```python
from build123d import *

# Parameters (mm, degrees)
F0_R     = 2.5
F0_R_2   = 8
F0_W     = 5
F0_H     = 9.9
F1_DEPTH = 3.5


with BuildPart() as f1:
    # F0 (on Top) → F1 (new body)
    with BuildSketch(Plane.XY):
        with BuildLine():
            ThreePointArc((0, -5), (-1.464466, -1.464466), (-5, 0))
            Line((-5, 0), (-125.9, 0))
            ThreePointArc((-125.9, 0), (-129.435534, -1.464466), (-130.9, -5))
            Line((-130.9, -5), (-130.9, -25))
            ThreePointArc((-130.9, -25), (-129.435534, -28.535534), (-125.9, -30))
            Line((-125.9, -30), (-5, -30))
            ThreePointArc((-5, -30), (-1.464466, -28.535534), (0, -25))
            Line((0, -25), (0, -5))
        make_face()
        with Locations((-96.3, -25.5)):
            Circle(F0_R, mode=Mode.SUBTRACT)
        with Locations((-76.3, -25.5)):
            Circle(F0_R, mode=Mode.SUBTRACT)
        with Locations((-56.3, -25.5)):
            Circle(F0_R, mode=Mode.SUBTRACT)
        with Locations((-36.3, -25.5)):
            Circle(F0_R, mode=Mode.SUBTRACT)
        with Locations((-16.3, -25.5)):
            Circle(F0_R, mode=Mode.SUBTRACT)
        with Locations((-118.9, -15)):
            Circle(F0_R_2, mode=Mode.SUBTRACT)
        with Locations((-104.4, -15)):
            Rectangle(F0_W, F0_H, mode=Mode.SUBTRACT)
        with Locations((-89.4, -14.965372)):
            Rectangle(F0_W, F0_H, mode=Mode.SUBTRACT)
        with Locations((-69.4, -14.965372)):
            Rectangle(F0_W, F0_H, mode=Mode.SUBTRACT)
        with Locations((-96.3, -4.5)):
            Circle(F0_R, mode=Mode.SUBTRACT)
        with Locations((-76.3, -4.5)):
            Circle(F0_R, mode=Mode.SUBTRACT)
        with Locations((-49.4, -14.965372)):
            Rectangle(F0_W, F0_H, mode=Mode.SUBTRACT)
        with Locations((-29.4, -14.965372)):
            Rectangle(F0_W, F0_H, mode=Mode.SUBTRACT)
        with Locations((-9.4, -14.965372)):
            Rectangle(F0_W, F0_H, mode=Mode.SUBTRACT)
        with Locations((-56.3, -4.5)):
            Circle(F0_R, mode=Mode.SUBTRACT)
        with Locations((-36.3, -4.5)):
            Circle(F0_R, mode=Mode.SUBTRACT)
        with Locations((-16.3, -4.5)):
            Circle(F0_R, mode=Mode.SUBTRACT)
    extrude(amount=F1_DEPTH)


solid = f1.part
```
Model file for the job. Use its own axes, mm. A direction names the side the tool comes from. Coordinates: 2 decimals unless noted, no trailing zeros. Order: outer loops, then holes, each group sorted by start corner. A loop starts at its lowest first (then second) coordinate and runs counter-clockwise, first axis right, second up. Notation, with made-up numbers: (18.5, 18.5) - (23.5, 18.5) arc R16 ccw to (23.5, 46.5) - close; hole circle Ø6 at (81.5, 68.5). An arc over 180 degrees is marked (long way). Return JSON: item names as keys, results as strings. Group by question number.
1) Tool access for faces 1 (the flat face through (-66, -15, 0)), 2 (the flat face through (-46.9, -15, 2)): list every direction of +Z, -Z, +X, -X, +Y, -Y with a clear straight run to the whole face (end or side of a thin tool).
2) Mould opens along Y. For faces 3 (the flat face through (-49, -10.015, 2)), 4 (the cylindrical face through (-129.47, -28.5, 1.73)), 5 (the flat face through (0, -15, 2)) say: released by +Y, released by -Y, zero draft, split by the parting line, or undercut.
3) Saw through at C-C, the plane x = -16.3. Write the cut outline in (y, z), plus the area to 3 significant figures.
4) Probe line 1 (Y direction, x = -36.3, z = 1.85); line 2 (Y direction, x = -89, z = 2.7); line 3 (Y direction, x = -119.5, z = 1.2). List the from-to ranges inside material, lowest first. Write a range as from..to.
5) Saw through at B-B, the plane y = -15. Count the separate pieces of the cut face and the enclosed holes in it, plus the area to 3 significant figures.
6) Saw through at A-A, the plane x = -118.9. Write the cut outline in (y, z).
Values found:
{
 "1": {"face 1": "-Z, +X, -X, +Y, -Y", "face 2": "+Z, -Z"},
 "2": {"face 3": "undercut", "face 4": "released by -Y", "face 5": "zero draft"},
 "3": {"outline": "(-30, 0) - (-28, 0) - (-28, 3.5) - (-30, 3.5) - close; (-23, 0) - (-7, 0) - (-7, 3.5) - (-23, 3.5) - close; (-2, 0) - (0, 0) - (0, 3.5) - (-2, 3.5) - close", "area": "70.0 mm²"},
 "4": {"line 1": "y = -30..-28, -23..-7, -2..0", "line 2": "y = -30..-19.92, -10.02..0", "line 3": "y = -30..-22.98, -7.02..0"},
 "5": {"separate pieces": "8", "enclosed holes": "0", "area": "297 mm²"},
 "6": {"outline": "(-30, 0) - (-23, 0) - (-23, 3.5) - (-30, 3.5) - close; (-7, 0) - (0, 0) - (0, 3.5) - (-7, 3.5) - close"}
}
